Design review of the part built by this model. Coordinates are the model's own, in mm. Round coordinates to 2 decimals unless told otherwise and drop trailing zeros. Loops run counter-clockwise (first coordinate to the right, second up) from the corner with the lowest first, then second, coordinate; pieces in that order, holes last. Notation, with made-up numbers: (-39, 76) -> (19, 76) arc R21 ccw to (19, 91) -> close; hole circle Ø11 at (69, 28.25). An arc over 180 degrees is marked (long way). Use a Markdown table: item, result. Add a question column.
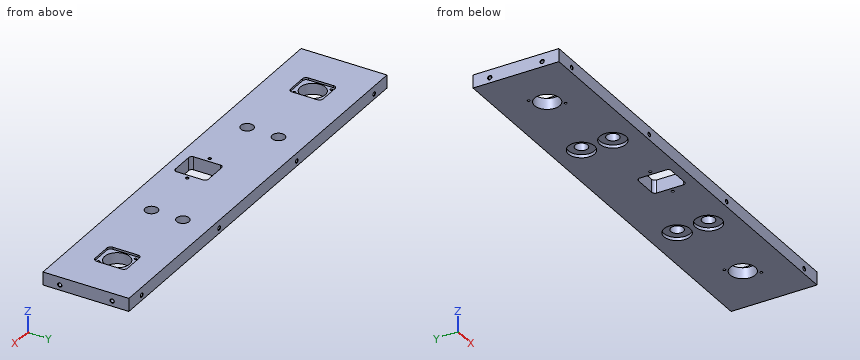
from build123d import *

# Parameters (mm, degrees)
SKETCH_1_W                   = 413
SKETCH_1_H                   = 82
EXTRUDE_1_DEPTH              = 12.5
SKETCH_2_R                   = 12
SKETCH_2_R_2                 = 6
SKETCH_2_W                   = 13.75
SKETCH_2_H                   = 31.5
CUT_EXTRUDE_1_DEPTH          = 13.5
HOLE_WIZARD_M3_1_D           = 2.5
HOLE_WIZARD_M3_1_CSINK_D     = 3.05
HOLE_WIZARD_M3_1_CSINK_ANGLE = 90
FILLET_1_R                   = 3
HOLE_WIZARD_M4_1_D           = 3.3
HOLE_WIZARD_M4_1_DEPTH       = 5
HOLE_WIZARD_M4_1_CSINK_D     = 4.05
HOLE_WIZARD_M4_1_CSINK_ANGLE = 90
HOLE_WIZARD_M4_1_TIP         = 0.991420021
HOLE_WIZARD_M4_2_D           = 3.3
HOLE_WIZARD_M4_2_DEPTH       = 5
HOLE_WIZARD_M4_2_CSINK_D     = 4.05
HOLE_WIZARD_M4_2_CSINK_ANGLE = 90
HOLE_WIZARD_M4_2_TIP         = 0.991420021
HOLE_WIZARD_M4_3_D           = 3.3
HOLE_WIZARD_M4_3_DEPTH       = 10.1
HOLE_WIZARD_M4_3_CSINK_D     = 4.05
HOLE_WIZARD_M4_3_CSINK_ANGLE = 90
HOLE_WIZARD_M4_3_TIP         = 0.991420021
HOLE_WIZARD_M4_4_D           = 3.3
HOLE_WIZARD_M4_4_DEPTH       = 10.1
HOLE_WIZARD_M4_4_CSINK_D     = 4.05
HOLE_WIZARD_M4_4_CSINK_ANGLE = 90
HOLE_WIZARD_M4_4_TIP         = 0.991420021
SKETCH_15_R                  = 12.5
CUT_EXTRUDE_2_DEPTH          = 3
SKETCH_16_W                  = 26
SKETCH_16_H                  = 31
CUT_EXTRUDE_3_DEPTH          = 2
FILLET_2_R                   = 3.5


with BuildPart() as part:
    # 草圖1 → 填料-伸長1 (new body)
    with BuildSketch(Plane.XY):
        with Locations((206.5, 41)):
            Rectangle(SKETCH_1_W, SKETCH_1_H)
    extrude(amount=EXTRUDE_1_DEPTH)

    # 草圖2 → 除料-伸長1 (cut, through all)
    with BuildSketch(Plane.XY.offset(12.5)):
        with Locations((50, 41)):
            Circle(SKETCH_2_R)
        with Locations((130, 56)):
            Circle(SKETCH_2_R_2)
        with Locations((130, 26)):
            Circle(SKETCH_2_R_2)
        with Locations((199.625, 25.25)):
            Rectangle(SKETCH_2_W, SKETCH_2_H)
        with Locations((213.375, 25.25)):
            Rectangle(SKETCH_2_W, SKETCH_2_H)
        with Locations((283, 56)):
            Circle(SKETCH_2_R_2)
        with Locations((283, 26)):
            Circle(SKETCH_2_R_2)
        with Locations((363, 41)):
            Circle(SKETCH_2_R)
    extrude(amount=-CUT_EXTRUDE_1_DEPTH, mode=Mode.SUBTRACT)

    # M3 螺紋孔1 (through all)
    with Locations(Plane.XY.offset(12.5)):
        with Locations((40.5, 53), (59.5, 29), (353.5, 53), (372.5, 29), (224.5, 25.25), (188.5, 25.25)):
            CounterSinkHole(HOLE_WIZARD_M3_1_D / 2, HOLE_WIZARD_M3_1_CSINK_D / 2, counter_sink_angle=HOLE_WIZARD_M3_1_CSINK_ANGLE)

    # 圓角1
    fillet_1_edges = [part.edges().sort_by_distance(p)[0] for p in [
        (192.75, 41, 6.25),
        (220.25, 41, 6.25),
        (220.25, 9.5, 6.25),
        (192.75, 9.5, 6.25),
    ]]
    fillet(fillet_1_edges, radius=FILLET_1_R)

    # M4 螺紋孔1
    with Locations(Plane(origin=(0, 82, 0), x_dir=(1, 0, 0), z_dir=(0, 1, 0))):
        with Locations((20.5, -5), (144.5, -5), (268.5, -5), (392.5, -5)):
            CounterSinkHole(HOLE_WIZARD_M4_1_D / 2, HOLE_WIZARD_M4_1_CSINK_D / 2, depth=HOLE_WIZARD_M4_1_DEPTH, counter_sink_angle=HOLE_WIZARD_M4_1_CSINK_ANGLE)
            with Locations((0, 0, -(HOLE_WIZARD_M4_1_DEPTH + HOLE_WIZARD_M4_1_TIP / 2))):  # 118° drill point
                Cone(0, HOLE_WIZARD_M4_1_D / 2, HOLE_WIZARD_M4_1_TIP, mode=Mode.SUBTRACT)

    # M4 螺紋孔2
    with Locations(Plane(origin=(0, 0, 0), x_dir=(-1, 0, 0), z_dir=(0, -1, 0))):
        with Locations((-144.5, -5), (-20.5, -5), (-268.5, -5), (-392.5, -5)):
            CounterSinkHole(HOLE_WIZARD_M4_2_D / 2, HOLE_WIZARD_M4_2_CSINK_D / 2, depth=HOLE_WIZARD_M4_2_DEPTH, counter_sink_angle=HOLE_WIZARD_M4_2_CSINK_ANGLE)
            with Locations((0, 0, -(HOLE_WIZARD_M4_2_DEPTH + HOLE_WIZARD_M4_2_TIP / 2))):  # 118° drill point
                Cone(0, HOLE_WIZARD_M4_2_D / 2, HOLE_WIZARD_M4_2_TIP, mode=Mode.SUBTRACT)

    # M4 螺紋孔3
    with Locations(Plane.ZY):
        with Locations((5, 66), (5, 16)):
            CounterSinkHole(HOLE_WIZARD_M4_3_D / 2, HOLE_WIZARD_M4_3_CSINK_D / 2, depth=HOLE_WIZARD_M4_3_DEPTH, counter_sink_angle=HOLE_WIZARD_M4_3_CSINK_ANGLE)
            with Locations((0, 0, -(HOLE_WIZARD_M4_3_DEPTH + HOLE_WIZARD_M4_3_TIP / 2))):  # 118° drill point
                Cone(0, HOLE_WIZARD_M4_3_D / 2, HOLE_WIZARD_M4_3_TIP, mode=Mode.SUBTRACT)

    # M4 螺紋孔4
    with Locations(Plane(origin=(413, 0, 0), x_dir=(0, 0, -1), z_dir=(1, 0, 0))):
        with Locations((-5, 66), (-5, 16)):
            CounterSinkHole(HOLE_WIZARD_M4_4_D / 2, HOLE_WIZARD_M4_4_CSINK_D / 2, depth=HOLE_WIZARD_M4_4_DEPTH, counter_sink_angle=HOLE_WIZARD_M4_4_CSINK_ANGLE)
            with Locations((0, 0, -(HOLE_WIZARD_M4_4_DEPTH + HOLE_WIZARD_M4_4_TIP / 2))):  # 118° drill point
                Cone(0, HOLE_WIZARD_M4_4_D / 2, HOLE_WIZARD_M4_4_TIP, mode=Mode.SUBTRACT)

    # 草圖15 → 除料-伸長2 (cut)
    with BuildSketch(Plane(origin=(0, 0, 0), x_dir=(-1, 0, 0), z_dir=(0, 0, -1))):
        with Locations((-283, 56)):
            Circle(SKETCH_15_R)
        with Locations((-283, 26)):
            Circle(SKETCH_15_R)
        with Locations((-130, 56)):
            Circle(SKETCH_15_R)
        with Locations((-130, 26)):
            Circle(SKETCH_15_R)
    extrude(amount=-CUT_EXTRUDE_2_DEPTH, mode=Mode.SUBTRACT)

    # 草圖16 → 除料-伸長3 (cut)
    with BuildSketch(Plane.XY.offset(12.5)):
        with Locations((50, 41)):
            Rectangle(SKETCH_16_W, SKETCH_16_H)
        with Locations((363, 41)):
            Rectangle(SKETCH_16_W, SKETCH_16_H)
    extrude(amount=-CUT_EXTRUDE_3_DEPTH, mode=Mode.SUBTRACT)

    # 圓角2
    fillet_2_edges = [part.edges().sort_by_distance(p)[0] for p in [
        (63, 56.5, 11.5),
        (63, 25.5, 11.5),
        (37, 25.5, 11.5),
        (37, 56.5, 11.5),
        (376, 56.5, 11.5),
        (376, 25.5, 11.5),
        (350, 25.5, 11.5),
        (350, 56.5, 11.5),
    ]]
    fillet(fillet_2_edges, radius=FILLET_2_R)


solid = part.part
1. Insertion check: P1, Ø4, axis at x = 144.5, z = 5, coming from the +Y side (3 decimals); P2, Ø2.5, axis at x = 392.5, z = 5, coming from the +Y side; P3, Ø7.5, axis at x = 278, y = 56, coming from the -Z side. Each pin has a flat end and moves straight along its axis. Give the tip position at first contact, or say it passes through.
2. To check wall thickness, follow probe 1 along X at (y, z) = (1.6, 5); probe 2 along Y at (x, z) = (130, 6.25); probe 3 along Y at (x, z) = (130, 1.25). State the ranges of each line that lie inside material, in increasing order. Write a range as from..to.
3. Consider section A-A on x = 283. State the section outline as (y, z) points.
Verdict:
| question | item | result |
|---|---|---|
| 1 | P1 | stops at y = 81.975 |
| 1 | P2 | stops at y = 76.76 |
| 1 | P3 | stops at z = 3 |
| 2 | probe 1 | x = 0..18.85, 22.15..142.85, 146.15..266.85, 270.15..390.85, 394.15..413 |
| 2 | probe 2 | y = 0..20, 32..50, 62..82 |
| 2 | probe 3 | y = 0..13.5, 38.5..43.5, 68.5..82 |
| 3 | outline | (0, 0) -> (13.5, 0) -> (13.5, 3) -> (20, 3) -> (20, 12.5) -> (0, 12.5) -> close; (32, 3) -> (38.5, 3) -> (38.5, 0) -> (43.5, 0) -> (43.5, 3) -> (50, 3) -> (50, 12.5) -> (32, 12.5) -> close; (62, 3) -> (68.5, 3) -> (68.5, 0) -> (82, 0) -> (82, 12.5) -> (62, 12.5) -> close |
